from build123d import *

# Parameters (mm, degrees)
BOSS_EXTRUDE1_DEPTH = 5.715


with BuildPart() as part:
    # Model → Boss-Extrude1 (new body)
    with BuildSketch(Plane.XY):
        Polygon((863.26218, 23.2006394), (875.52784, 23.2006394), (875.52784, 28.91536), (886.95784, 28.91536), (886.95784, 23.2006394), (898.38784, 23.2006394), (898.38784, 28.91536), (909.81784, 28.91536), (909.81784, 23.2006394), (922.08096, 23.2006394), (922.08096, 279.63114), (909.81784, 279.63114), (909.81784, 273.91614), (898.38784, 273.91614), (898.38784, 279.63114), (886.95784, 279.63114), (886.95784, 273.91614), (875.52784, 273.91614), (875.52784, 279.63114), (863.26218, 279.63114), (863.26218, 251.055124), (863.26218, 250.316746), (863.64826, 248.098056), (864.54234, 245.775988), (864.79126, 245.340378), (865.04272, 244.906546), (866.6099, 242.974368), (868.54284, 241.407696), (868.97718, 241.156744), (869.40898, 240.906046), (871.34446, 239.34039), (872.9091, 237.408466), (873.16056, 236.972856), (873.41202, 236.539024), (874.30356, 234.216956), (874.69472, 231.998266), (874.69472, 231.25811), (874.69472, 71.572628), (874.69218, 71.070978), (874.30356, 68.615306), (873.41202, 66.293238), (873.16056, 65.857882), (872.9091, 65.423796), (871.34446, 63.491872), (869.40898, 61.924946), (868.97718, 61.673994), (868.54284, 61.423296), (866.6099, 59.857894), (865.04272, 57.925716), (864.79126, 57.49036), (864.54234, 57.056274), (863.64826, 54.734206), (863.26218, 52.515516), (863.26218, 51.775868), align=None)
        Polygon((880.40718, 254.28448), (880.40718, 259.99948), (886.12218, 259.99948), (886.12218, 248.570496), (880.40718, 248.570496), align=None, mode=Mode.SUBTRACT)
        Polygon((880.40718, 231.424988), (880.40718, 237.141004), (886.12218, 237.141004), (886.12218, 225.710496), (880.40718, 225.710496), align=None, mode=Mode.SUBTRACT)
        Polygon((880.40718, 208.566004), (880.40718, 214.28075), (886.12218, 214.28075), (886.12218, 202.849988), (880.40718, 202.849988), align=None, mode=Mode.SUBTRACT)
        Polygon((880.40718, 185.70575), (880.40718, 191.420496), (886.12218, 191.420496), (886.12218, 179.991004), (880.40718, 179.991004), align=None, mode=Mode.SUBTRACT)
        Polygon((880.40718, 162.845496), (880.40718, 168.560496), (886.12218, 168.560496), (886.12218, 157.13075), (880.40718, 157.13075), align=None, mode=Mode.SUBTRACT)
        Polygon((880.40718, 139.985496), (880.40718, 145.699988), (886.12218, 145.699988), (886.12218, 134.270496), (880.40718, 134.270496), align=None, mode=Mode.SUBTRACT)
        Polygon((880.40718, 117.124988), (880.40718, 122.841004), (886.12218, 122.841004), (886.12218, 111.410496), (880.40718, 111.410496), align=None, mode=Mode.SUBTRACT)
        Polygon((880.40718, 94.266004), (880.40718, 99.98075), (886.12218, 99.98075), (886.12218, 88.549988), (880.40718, 88.549988), align=None, mode=Mode.SUBTRACT)
        Polygon((880.40718, 71.40575), (880.40718, 77.120496), (886.12218, 77.120496), (886.12218, 65.691004), (880.40718, 65.691004), align=None, mode=Mode.SUBTRACT)
        Polygon((880.40718, 48.545496), (880.40718, 54.260496), (886.12218, 54.260496), (886.12218, 42.83075), (880.40718, 42.83075), align=None, mode=Mode.SUBTRACT)
    extrude(amount=BOSS_EXTRUDE1_DEPTH)


solid = part.part
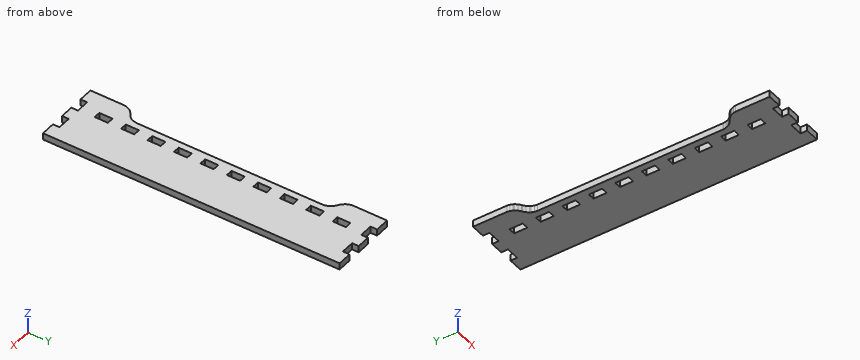
CAD build for the part. Positions are in the model's coordinates, mm. Coordinates: 2 decimals unless noted, no trailing zeros. Loops run counter-clockwise (first coordinate to the right, second up) from the corner with the lowest first, then second, coordinate; pieces in that order, holes last. Notation, with made-up numbers: (29, 70.25) - (47, 70.25) arc R21 ccw to (47, 98.25) - close; hole circle Ø6 at (47.25, 6.25). An arc over 180 degrees is marked (long way). Use one line per item in the form item = value. Start each with the question number.
1) Band-saw the part on D-D (x = 901). Give the cut face in (y, z) (3 decimals), and give its area (3 significant figures).
2) Drill centre lines: L1, parallel to X at y = 212.5, z = 2.8; L2, parallel to Y at x = 869, z = 0.55; L3, parallel to Y at x = 906, z = 2.15. Where is each one in solid material? Low to high. Write a range as from..to.
3) Band-saw the part on B-B (x = 883). State how many separate pieces and enclosed holes the cut face has, and give its area (3 significant figures).
4) Flat gauge pins, fed straight in: pin 1 (1 mm diameter, centred on x = 872.5, y = 185.5, fed in from +Z); pin 2 (3 mm diameter, centred on x = 882.5, z = 2, fed in from -Y); pin 3 (1.7 mm diameter, centred on x = 883, z = 2, fed in from +Y). Where does each tip first touch, or does it go through?
5) Band-saw the part on A-A (y = 97.5). Give the cut face in (x, z) (3 decimals), and give its area (3 significant figures).
Check values:
q1.outline = (28.915, 0) - (273.916, 0) - (273.916, 5.715) - (28.915, 5.715) - close
q1.area = 1,400 mm2
q2.L1 = 874.69..880.41, 886.12..922.08
q2.L2 = 23.2..61.69, 241.14..279.63
q2.L3 = 28.92..273.92
q3.separate_pieces = 11
q3.enclosed_holes = 0
q3.area = 747 mm2
q4.pin_1 = through
q4.pin_2 = 28.92
q4.pin_3 = 273.92
q5.outline = (874.695, 0) - (880.407, 0) - (880.407, 5.715) - (874.695, 5.715) - close; (886.122, 0) - (922.081, 0) - (922.081, 5.715) - (886.122, 5.715) - close
q5.area = 238 mm2
